For this review, take the finished solid that the model builds, in its own axes (mm). Face numbers are marked on the shaded views. A direction names the side the tool comes from. Give positions to 0.01 mm unless a question says otherwise; leave off trailing zeros. Order: outer loops, then holes, each group sorted by start corner. A loop starts at its lowest first (then second) coordinate and runs counter-clockwise, first axis right, second up. Notation, with made-up numbers: (-38.5, 59.25) -> (-9.5, 59.25) arc R25 cw to (-9.5, 84.25) -> close; hole circle Ø9 at (-11, -34). An arc over 180 degrees is marked (long way). Return JSON: item names as keys, results as strings. Group by question number.
1) To check wall thickness, follow line 1 along X through (y, z) = (1.2, 0); line 2 along X through (y, z) = (-0.75, 8); line 3 along Z through (x, y) = (-10, -1.5). State the ranges of each line that lie inside material, in increasing order.
2) Add section A-A (z = 0). Give the boundary of the cut face in (x, y).
3) Add section D-D (z = -6.5). Give the boundary of the cut face in (x, y), then the cut area to 3 significant figures.
4) For the marked faces 1, 2 and 3, list the 3-axis set-ups (+Z, -Z, +X, -X, +Y, -Y) from which the entire face can be reached by the end or side of a thin tool; tool diameter is ignored.
5) The part is to be moulded in two halves that separate along X. For the marked faces 4, 5 and 6, say which applies: released by +X, released by -X, zero draft, split by the parting line, or undercut.
6) Insertion check: P1, Ø5.5, axis at x = 0, z = 0, coming from the -Y side; P2, Ø1.6, axis at y = -2, z = -1, coming from the +X side; P3, Ø3, axis at x = -9.83, z = -6.88, coming from the -Y side; P4, Ø1.5, axis at x = 12.5, y = 0.5, coming from the -Z side. Each pin has a flat end and moves straight along its axis. Give the tip position at first contact, or say it passes through.
7) Add section C-C (y = -3). Give the boundary of the cut face in (x, z).
from build123d import *
from build123d.topology import SkipClean

# Parameters (mm, degrees)
SKETCH_1_R          = 14
SKETCH_1_R_2        = 2.1
EXTRUDE_1_DEPTH     = 3
EXTRUDE_START       = 1.6
SKETCH_3_R          = 17.5
SKETCH_3_R_2        = 2.1
EXTRUDE_2_DEPTH     = 1.6
EXTRUDE_START_2     = 2
EXTRUDE_5_DEPTH     = 2
SKETCH_8_R          = 1.6
CUT_EXTRUDE_2_DEPTH = 26.613668226


with BuildPart() as part:
    # ｽｹｯﾁ1 → ﾎﾞｽ - 押し出し1 (new body)
    with BuildSketch(Plane(origin=(0, 0, 0), x_dir=(1, 0, 0), z_dir=(0, 1, 0))):
        with Locations(Location((0, 0, 0), (0, 0, 270))):
            Circle(SKETCH_1_R)
        with Locations(Location((0, 0, 0), (0, 0, 270))):
            Circle(SKETCH_1_R_2, mode=Mode.SUBTRACT)
    extrude(amount=EXTRUDE_1_DEPTH)

    # ｽｹｯﾁ3 → ﾎﾞｽ - 押し出し2 (add)
    with SkipClean():  # the faces are left unmerged after this step: merging them gives an invalid solid
        with BuildSketch(Plane.XZ.offset(EXTRUDE_START)):
            with Locations(Location((0, 0, 0), (0, 0, 270))):
                Circle(SKETCH_3_R)
            with Locations(Location((0, 0, 0), (0, 0, 270))):
                Circle(SKETCH_3_R_2, mode=Mode.SUBTRACT)
        extrude(amount=-EXTRUDE_2_DEPTH)

    # ｽｹｯﾁ7 → ﾎﾞｽ - 押し出し5 (add)
    with BuildSketch(Plane.XZ.offset(1.6).offset(EXTRUDE_START_2)):
        with BuildLine():
            Line((-6, 16.439282223), (-6, -16.439282223))
            ThreePointArc((-6, -16.439282223), (-17.5, 0), (-6, 16.439282223))
        make_face()
        with BuildLine():
            Line((6, 16.439282223), (6, -16.439282223))
            ThreePointArc((6, -16.439282223), (17.5, 0), (6, 16.439282223))
        make_face()
    extrude(amount=-EXTRUDE_5_DEPTH)

    # ｽｹｯﾁ8 → ｶｯﾄ - 押し出し2 (cut, through all)
    with BuildSketch(Plane.XZ.offset(3.6)):
        with Locations(Location((9.829824531, 6.882917236, 0), (0, 0, 270))):
            Circle(SKETCH_8_R)
        with Locations(Location((-9.829824531, -6.882917236, 0), (0, 0, 90))):
            Circle(SKETCH_8_R)
        with Locations(Location((-9.829824531, 6.882917236, 0), (0, 0, 270))):
            Circle(SKETCH_8_R)
        with Locations(Location((9.829824531, -6.882917236, 0), (0, 0, 270))):
            Circle(SKETCH_8_R)
    extrude(amount=-CUT_EXTRUDE_2_DEPTH, mode=Mode.SUBTRACT)


solid = part.part
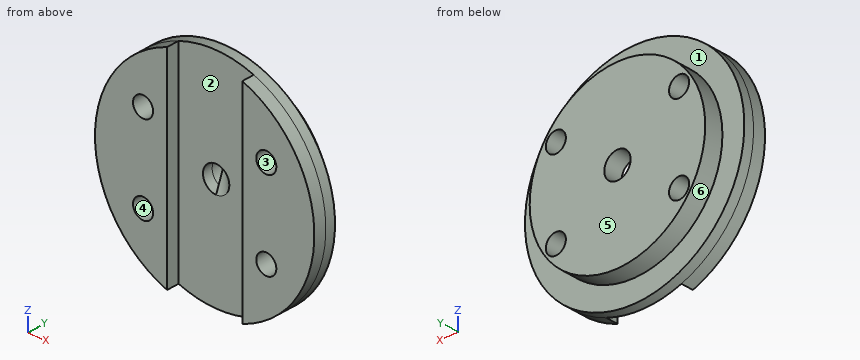
Evaluation:
{
 "1": {"line 1": "-14 to -2.1, 2.1 to 14", "line 2": "-15.56 to -10.98, -8.68 to 8.68, 10.98 to 15.56", "line 3": "-14.36 to -8.47, -5.29 to 5.29, 8.47 to 14.36"},
 "2": {"outline": "(-17.5, -3.6) -> (-6, -3.6) -> (-6, -1.6) -> (-2.1, -1.6) -> (-2.1, 3) -> (-14, 3) -> (-14, 0) -> (-17.5, 0) -> close; (2.1, -1.6) -> (6, -1.6) -> (6, -3.6) -> (17.5, -3.6) -> (17.5, 0) -> (14, 0) -> (14, 3) -> (2.1, 3) -> close"},
 "3": {"outline": "(-16.25, -3.6) -> (-11.38, -3.6) -> (-11.38, 3) -> (-12.4, 3) -> (-12.4, 0) -> (-16.25, 0) -> close; (-8.28, -3.6) -> (-6, -3.6) -> (-6, -1.6) -> (6, -1.6) -> (6, -3.6) -> (8.28, -3.6) -> (8.28, 3) -> (-8.28, 3) -> close; (11.38, -3.6) -> (16.25, -3.6) -> (16.25, 0) -> (12.4, 0) -> (12.4, 3) -> (11.38, 3) -> close", "area": "126 mm^2"},
 "4": {"face 1": "+Y", "face 2": "+Z, -Z, -Y", "face 3": "+Y, -Y"},
 "5": {"face 4": "undercut", "face 5": "zero draft", "face 6": "split by the parting line"},
 "6": {"P1": "y = -1.6", "P2": "x = 17.5", "P3": "through", "P4": "z = -12.79"},
 "7": {"outline": "(-6, -16.44) -> (-6, 16.44) arc R17.5 ccw to start; (6, -16.44) arc R17.5 ccw to (6, 16.44) -> close; hole circle Ø3.2 at (-9.83, -6.88); hole circle Ø3.2 at (-9.83, 6.88); hole circle Ø3.2 at (9.83, -6.88); hole circle Ø3.2 at (9.83, 6.88)"}
}
